from build123d import *

# Parameters (mm, degrees)
F0_W     = 35.56
F0_H     = 17.78
F1_DEPTH = 1.57
F2_W     = 4.36
F2_H     = 3.75
F3_DEPTH = 3.07
F2_W_2   = 2.2
F2_H_2   = 1.5
F4_DEPTH = 2.5


with BuildPart() as f1:
    # F0 (on Top) → F1 (new body)
    with BuildSketch(Plane.XY):
        Rectangle(F0_W, F0_H)
    extrude(amount=F1_DEPTH)

    # F2 (on face) → F3 (join)
    with BuildSketch(Plane.XY.offset(1.57)):
        with Locations((-15.6, 1.875)):
            Rectangle(F2_W, F2_H)
        Polygon((-17.78, -3.75), (-17.78, 0), (-17.78, 3.75), (-18.48, 3.75), (-18.48, -3.75), align=None)
        with Locations((-15.6, -1.875)):
            Rectangle(F2_W, F2_H)
    extrude(amount=F3_DEPTH)

    # F2 (on face) → F4 (join)
    with BuildSketch(Plane.XY.offset(1.57)):
        with Locations((13.841648, 0.75)):
            Rectangle(F2_W_2, F2_H_2)
        with Locations((13.841648, -0.75)):
            Rectangle(F2_W_2, F2_H_2)
    extrude(amount=F4_DEPTH)


solid = f1.part
The model under review builds one solid part; all positions refer to its coordinate system, in mm. A direction names the side the tool comes from. Round coordinates to 2 decimals unless told otherwise and drop trailing zeros. Write each loop counter-clockwise with the first axis right and the second up, starting at its lowest first coordinate (ties: lowest second). Pieces come first, ordered by that corner, then holes. Notation, with made-up numbers: M 82,-16 L 103,-16 A24 ccw 103,8 Z; hole C 35.5,67 d2. An arc over 180 degrees is marked long. Answer as CSV lines item,"result". Start each with the question number.
Q1. Wall thickness on line 1 along X through (y, z) = (0.25, 1.6); line 2 along X through (y, z) = (-4, 1.45); line 3 along Z through (x, y) = (-10, 0.5): over which ranges is each line inside the solid? List them lowest first.
Q2. Clearance check with flat-ended pins moving along their axes: P1, Ø1.8, axis at x = 13.5, z = 3, coming from the +Y side; P2, Ø8, axis at x = -3, y = -3, coming from the +Z side; P3, Ø1.3, axis at y = -3.5, z = 0.5, coming from the -X side; P4, Ø8, axis at x = 1.5, y = -3, coming from the -Z side. State where each tip first meets the part, or that it passes through.
Q3. Tool access review of faces 1 (the face through (14, -1.5, 3)), 2 (the face through (-16, 3.75, 3)), 3 (the face through (14.942, 0, 3)): name each direction out of +Z, -Z, +X, -X, +Y, -Y from which nothing blocks a thin tool from reaching the whole face with its end or side.
Q4. Consider section B-B, the plane y = -5.5. Give the boundary of the cut face in (x, z).
Q5. Consider section C-C, the plane x = -2.5. Give the boundary of the cut face in (y, z), then the cut area to 3 significant figures.
Q6. The part is to be moulded in two halves that separate along X. For faces 4 (the face through (-17.78, 0, 1)), 5 (the face through (-16, -3.75, 3)), 6 (the face through (-13.42, 0, 3)), say which applies: +X half, -X half, draft (parallel to the pull), parting line (faces both ways), or undercut.
Q7. Consider section A-A, the plane z = 3.1. Give the boundary of the cut face in (x, y).
Result set:
1,line 1,"x = -18.48 to -13.42, 12.74 to 14.94"
1,line 2,"x = -17.78 to 17.78"
1,line 3,"z = 0 to 1.57"
2,P1,"stops at y = 1.5"
2,P2,"stops at z = 1.57"
2,P3,"stops at x = -17.78"
2,P4,"stops at z = 0"
3,face 1,"+Z, +X, -Y"
3,face 2,"+Z, +X, -X, +Y"
3,face 3,"+Z, +X, +Y, -Y"
4,outline,"M -17.78,0 L 17.78,0 L 17.78,1.57 L -17.78,1.57 Z"
5,outline,"M -8.89,0 L 8.89,0 L 8.89,1.57 L -8.89,1.57 Z"
5,area,"27.9 mm²"
6,face 4,"-X half"
6,face 5,"draft"
6,face 6,"undercut"
7,outline,"M -18.48,-3.75 L -13.42,-3.75 L -13.42,3.75 L -18.48,3.75 Z; M 12.74,-1.5 L 14.94,-1.5 L 14.94,1.5 L 12.74,1.5 Z"
